```python
from build123d import *

# Parameters (mm, degrees)
F1_DEPTH = 12.7
F2_R     = 4.6763821429
F3_R     = 0.12308652
F5_D     = 8.89


with BuildPart() as f1:
    # F0 (on Top) → F1 (new body)
    with BuildSketch(Plane.XY):
        Polygon((-64.9482621324, 50.8), (-71.2982621324, 50.8), (-71.2982621324, 0), (-53.2793551183, -17.9019269917), (-40.4947772622, -17.9019269917), (-22.5928502705, 0.1169800224), (-36.5162245659, 0), (-43.3580465615, -6.8865298358), (-58.0167323134, -6.8865298358), (-64.9482621324, 0), align=None)
    extrude(amount=F1_DEPTH)

    # F2
    f2_edges = [f1.edges().sort_by_distance(p)[0] for p in [
        (-22.59285, 0.11698, 6.35),
    ]]
    fillet(f2_edges, radius=F2_R)

    # F3
    f3_edges = [f1.edges().sort_by_distance(p)[0] for p in [
        (-33.964892, 0.021436, 6.35),
        (-36.516225, 0, 6.35),
    ]]
    fillet(f3_edges, radius=F3_R)

    # F5 (through all)
    with Locations(Plane.YZ):
        with Locations((39.1929335892, 6.155018229)):
            Hole(F5_D / 2)


solid = f1.part
```
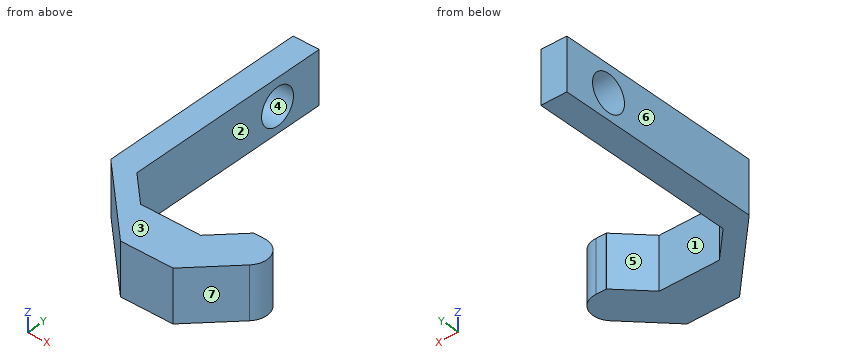
Work out the finished part from the listing and answer in its coordinate system (mm). Face numbers are marked on the shaded views. A direction names the side the tool comes from. Give positions to 0.01 mm unless a question says otherwise; leave off trailing zeros. Write each loop counter-clockwise with the first axis right and the second up, starting at its lowest first coordinate (ties: lowest second). Pieces come first, ordered by that corner, then holes.
(1) The part is cut by section A-A on y = -3. Write down the section's boundary in (x, z), plus the area to 3 significant figures.
Final values:
outline: (-68.28, 0) - (-61.93, 0) - (-61.93, 12.7) - (-68.28, 12.7) - close; (-39.5, 0) - (-29.55, 0) - (-29.55, 12.7) - (-39.5, 12.7) - close
area: 207 mm2
(2) The part is cut by section D-D on x = -49. Write down the section's boundary in (y, z), plus the area to 3 significant figures.
Final values:
outline: (-17.9, 0) - (-6.89, 0) - (-6.89, 12.7) - (-17.9, 12.7) - close
area: 140 mm2
(3) Flat-ended cylindrical pins translate along their axes: pin 1 Ø2 at (x, y) = (-40.5, -2.5) entering from -Z; pin 2 Ø6 at (x, z) = (-64, 5.5) entering from -Y; pin 3 Ø1.5 at (x, z) = (-51.5, 2.5) entering from +Y. Find the tip coordinate at first contact, or state that the pin passes through.
Final values:
pin 1: passes through
pin 2: stops at y = -10.23
pin 3: stops at y = -6.89
(4) Which of the six approach directions +Z, -Z, +X, -X, +Y, -Y give full straight-line access (tool end or side, diameter ignored) to the marked faces 1, 2 and 3?
Final values:
face 1: +Z, -Z, +Y
face 2: +Z, -Z, +X, +Y
face 3: +Z, +X, -X, +Y, -Y
(5) The part is cut by section B-B on z = 5. Write down the section's boundary in (x, y), plus the area to 3 significant figures.
Final values:
outline: (-71.3, 0) - (-53.28, -17.9) - (-40.49, -17.9) - (-30.61, -7.95) arc R4.68 ccw to (-33.96, 0.02) - (-36.47, 0) arc R0.12 ccw to (-36.55, -0.04) - (-43.36, -6.89) - (-58.02, -6.89) - (-64.95, 0) - (-64.95, 34.9) - (-71.3, 34.9) - close; (-71.3, 43.49) - (-64.95, 43.49) - (-64.95, 50.8) - (-71.3, 50.8) - close
area: 642 mm2
(6) Straight lines are drawn through the part: line 1 (X direction, y = 32.5, z = 7.5); line 2 (Y direction, x = -50.5, z = 9.25); line 3 (Y direction, x = -65, z = 8). For each, find the intervals that lie inside material, in ascending order.
Final values:
line 1: x = -71.3 to -64.95
line 2: y = -17.9 to -6.89
line 3: y = -6.26 to 35.15, 43.24 to 50.8
(7) The part is cut by section C-C on y = 8.5. Write down the section's boundary in (x, z), plus the area to 3 significant figures.
Final values:
outline: (-71.3, 0) - (-64.95, 0) - (-64.95, 12.7) - (-71.3, 12.7) - close
area: 80.6 mm2
(8) The mould has two halves that part along Y. Classify the marked faces 4, 5, 6 and 7: pulls with the +Y half, pulls with the -Y half, needs draft (parallel to the pull), parting line crosses it, or undercut.
Final values:
face 4: undercut
face 5: pulls with the +Y half
face 6: needs draft
face 7: pulls with the -Y half
